Build history of the part. All positions in model axes, mm. A direction names the side the tool comes from. Round coordinates to 2 decimals unless told otherwise and drop trailing zeros. Write each loop counter-clockwise with the first axis right and the second up, starting at its lowest first coordinate (ties: lowest second). Pieces come first, ordered by that corner, then holes. Notation, with made-up numbers: (-29, 68.25) -> (-21, 68.25) arc R7 ccw to (-21, 74.25) -> close; hole circle Ø11 at (86.25, -32). An arc over 180 degrees is marked (long way). Answer in a Markdown table with one row per item.
```python
from build123d import *

# Parameters (mm, degrees)
SKETCH2_R          = 12.718
CUT_EXTRUDE1_DEPTH = 82.74
SKETCH3_R          = 10
CUT_EXTRUDE2_DEPTH = 79.507
SKETCH4_W          = 1.691
SKETCH4_H          = 6.375
CUT_EXTRUDE3_DEPTH = 56


with BuildPart() as part:
    # Sketch1 → Revolve1 (revolve)
    with BuildSketch(Plane.XY, mode=Mode.PRIVATE) as revolve1_sk:
        with BuildLine():
            Line((-80.911998208, 0), (-80.911998208, 12.718))
            Line((-80.911998208, 12.718), (-70.911998208, 12.718))
            Line((-70.911998208, 12.718), (-70.911998208, 32.718))
            add(Edge.make_bspline(
                [(-70.911998208, 32.718), (-72.296532146, 50.185235542), (-58.681197048, 63.170292577), (-38.636582778, 76.893357171), (-26.258344783, 86.831311493), (-12.152126662, 86.899446164), (-6.607628807, 90)],
                knots=[0, 0, 0, 0, 0.504233074, 0.563304469, 0.79660287, 1, 1, 1, 1], degree=3))
            Line((-6.607628807, 90), (-1.664998208, 90))
            Line((-1.664998208, 90), (-1.664998208, 93))
            Line((-1.664998208, 93), (4.335001792, 93))
            Line((4.335001792, 93), (23.827899809, 15))
            Line((23.827899809, 15), (48.827899809, 15))
            Line((48.827899809, 15), (64.335001792, 91.202154094))
            Line((64.335001792, 91.202154094), (74.335001792, 91.202154094))
            Line((74.335001792, 91.202154094), (74.335001792, 14.709294291))
            Line((74.335001792, 14.709294291), (79.335001792, 14.709294291))
            Line((79.335001792, 14.709294291), (79.335001792, 0))
            Line((79.335001792, 0), (-80.911998208, 0))
        make_face()
    revolve(revolve1_sk.sketch.rotate(Axis((-81.835688806, 0, 0), (1, 0, 0)), 90), axis=Axis((-81.835688806, 0, 0), (1, 0, 0)))

    # Sketch2 → Cut-Extrude1 (cut)
    with BuildSketch(Plane(origin=(79.335001792, 0, 0), x_dir=(0, 0, -1), z_dir=(1, 0, 0))):
        with Locations(Location((0, 0, 0), (0, 0, 180))):
            Circle(SKETCH2_R)
    extrude(amount=-CUT_EXTRUDE1_DEPTH, mode=Mode.SUBTRACT)

    # Sketch3 → Cut-Extrude2 (cut)
    with BuildSketch(Plane.ZY.offset(80.911998208)):
        Circle(SKETCH3_R)
    extrude(amount=-CUT_EXTRUDE2_DEPTH, mode=Mode.SUBTRACT)

    # Chamfer1
    # the kernel refuses this chamfer: 3, 1.732050808 mm, written as the material it takes off along each edge
    with BuildSketch(Plane(origin=(-3.404998208, 0, 0), x_dir=(0, 0, 1), z_dir=(0, -1, 0))) as chamfer1_piece_1_section:
        with BuildLine():
            Line((9.896076952, 1.792050808), (13.103923048, -0.06))
            Line((13.103923048, -0.06), (13.103923048, -0.12))
            ThreePointArc((13.103923048, -0.12), (11.551961524, -0.06), (10, -0.06))
            Line((10, -0.06), (9.94, 0))
            ThreePointArc((9.94, 0), (9.94, 0.896025404), (9.836076952, 1.792050808))
            Line((9.836076952, 1.792050808), (9.896076952, 1.792050808))
        make_face()
    chamfer1_piece_1 = revolve(axis=Axis((-3.404998208, 0, 0), (-1, 0, 0)), mode=Mode.PRIVATE)
    chamfer1_piece_1 = chamfer1_piece_1 & Plane(origin=(-4.331873762, 0, 0), x_dir=(0, 0, 1), z_dir=(1, 0, 0)) * Cylinder(12.718, 53, mode=Mode.PRIVATE)
    add(chamfer1_piece_1, mode=Mode.SUBTRACT)

    # Sketch4 → Cut-Extrude3 (cut)
    with BuildSketch(Plane(origin=(79.335001792, 0, 0), x_dir=(0, 0, -1), z_dir=(1, 0, 0))):
        with Locations((12.718, 0)):
            Rectangle(SKETCH4_W, SKETCH4_H)
    extrude(amount=-CUT_EXTRUDE3_DEPTH, mode=Mode.SUBTRACT)


solid = part.part
```
Q1. Saw through at A-A on x = 8.5. Write the cut outline in (y, z), plus the area to 3 significant figures.
A:
| item | result |
|---|---|
| outline | circle Ø152.67 at (0, 0); hole circle Ø25.44 at (0, 0) |
| area | 17,800 mm² |
Q2. Drop flat-ended pins along their axis: P1, Ø4, axis at y = 71, z = 49, coming from the +X side (3 decimals); P2, Ø16, axis at y = 0, z = 0, coming from the +X side; P3, Ø1.9, axis at x = 45.5, y = -1.5, coming from the +Z side; P4, Ø2, axis at x = -22.5, y = -13, coming from the -Z side. Give the stop position or say it passes through.
A:
| item | result |
|---|---|
| P1 | x = 74.335 |
| P2 | through |
| P3 | z = 14.99 |
| P4 | z = -84.85 |
Q3. Two-plate mould, pull along Z, no slides. Class faces 1 (the cylindrical face through (-43.55, 3, 9.54)), 2 (the flat face through (74.335, 19, -1)), 3 (the cylindrical face through (76.87, 8.95, -11.673)): released by +Z, released by -Z, zero draft, split by the parting line, or undercut.
A:
| item | result |
|---|---|
| face 1 | undercut |
| face 2 | zero draft |
| face 3 | split by the parting line |
Q4. Which spindle directions (+Z, -Z, +X, -X, +Y, -Y) get a long thin tool onto all of the face, cutting with end or side? Do faces 4 (the conical face through (22.88, 16.67, 8.67)), 5 (the cylindrical face through (69.405, -90.426, -11.873)), 6 (the cylindrical face through (-4.102, 79.845, 41.53)), 7 (the flat face through (79.335, -12.1, -4.4)). Say none if no direction does.
A:
| item | result |
|---|---|
| face 4 | none |
| face 5 | +X |
| face 6 | -X |
| face 7 | +Z, -Z, +X, +Y, -Y |
Q5. Wall check: line 1 (Y direction, x = 46.5, z = 0); line 2 (X direction, y = 36.5, z = -9) (3 decimals); line 3 (X direction, y = -52.5, z = 7) (3 decimals). Give the ranges that are in metal, low to high. Write a range as [from, to].
A:
| item | result |
|---|---|
| line 1 | [-15, -12.72], [12.72, 15] |
| line 2 | [-70.947, 18.182], [53.426, 74.335] |
| line 3 | [-65.781, 14.34], [56.554, 74.335] |
